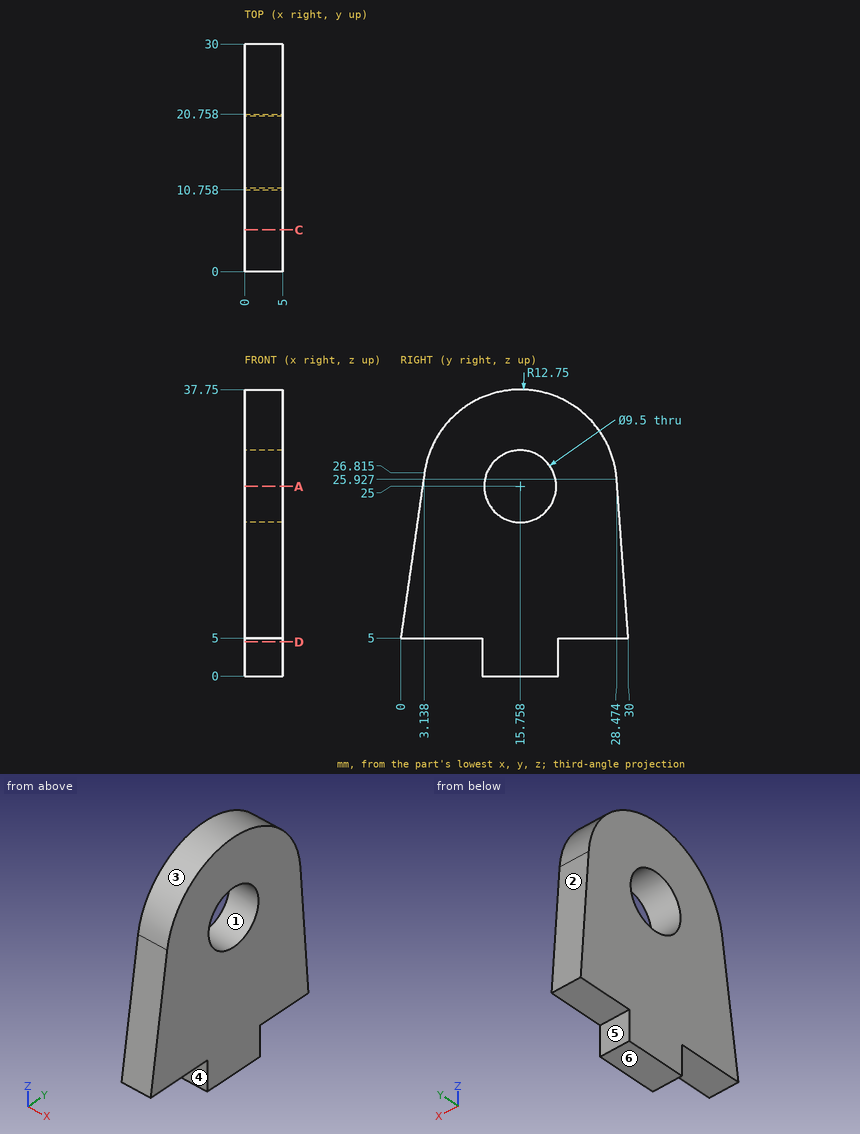
Print and shaded views of the part. All mm, measured from the part's lowest x, y and z. A direction names the side the tool comes from. Round coordinates to 2 decimals unless told otherwise and drop trailing zeros. Write each loop counter-clockwise with the first axis right and the second up, starting at its lowest first coordinate (ties: lowest second). Pieces come first, ordered by that corner, then holes. Notation, with made-up numbers: (-7.5, 63) -> (42.5, 63) arc R16 cw to (42.5, 76) -> close; hole circle Ø2 at (-14, 46.5). An arc over 180 degrees is marked (long way). Write item = value, one per line.
(1) Tool access for the marked faces 4, 5 and 6: list every direction of +Z, -Z, +X, -X, +Y, -Y with a clear straight run to the whole face (end or side of a thin tool).
Answer:
face_4 = -Z, +X, -X, -Y
face_5 = -Z, +X, -X, +Y
face_6 = -Z, +X, -X, +Y, -Y
(2) Two-plate mould, pull along Y, no slides. Class the marked faces 1, 2 and 3: pulls with the +Y half, pulls with the -Y half, needs draft (parallel to the pull), parting line crosses it, or undercut.
Answer:
face_1 = undercut
face_2 = pulls with the +Y half
face_3 = parting line crosses it
(3) Probe L1, parallel to Y at x = 4.2, z = 2; L2, parallel to Y at x = 1.3, z = 25; L3, parallel to Z at x = 1.15, y = 13. List the from-to ranges inside material, lowest first.
Answer:
L1 = 10.76 to 20.76
L2 = 2.88 to 11.01, 20.51 to 28.54
L3 = 0 to 21.13, 28.87 to 37.45
(4) Band-saw the part on C-C (y = 5.5). Give the cut face in (x, z).
Answer:
outline = (0, 5) -> (5, 5) -> (5, 32.57) -> (0, 32.57) -> close
(5) Band-saw the part on D-D (z = 4.5). Give the cut face in (x, y).
Answer:
outline = (0, 10.76) -> (5, 10.76) -> (5, 20.76) -> (0, 20.76) -> close
(6) Band-saw the part on A-A (z = 25). Give the cut face in (x, y).
Answer:
outline = (0, 2.88) -> (5, 2.88) -> (5, 11.01) -> (0, 11.01) -> close; (0, 20.51) -> (5, 20.51) -> (5, 28.54) -> (0, 28.54) -> close
(7) Flat gauge pins, fed straight in: pin 1 (12.5 mm diameter, centred on y = 15.76, z = 25, fed in from -X); pin 2 (1 mm diameter, centred on x = 0.5, y = 16.5, fed in from +Z); pin 3 (1 mm diameter, centred on x = 1.5, z = 30, fed in from +Y); pin 4 (2.5 mm diameter, centred on x = 3.5, z = 2, fed in from +Y). Where does each tip first touch, or does it go through?
Answer:
pin_1 = 0
pin_2 = 37.75
pin_3 = 27.69
pin_4 = 20.76
